Autodesk Inventor part; units mm, degrees
ref_plane "YZ Plane" through (0, 0, 0) normal (1, 0, 0) x (0, 1, 0)
ref_plane "XZ Plane" through (0, 0, 0) normal (0, 1, 0) x (-1, 0, 0)
ref_plane "XY Plane" through (0, 0, 0) normal (0, 0, 1) x (1, 0, 0)
sketch "Esboço1" plane through (0, 0, 0) normal (0, 1, 0) x (-1, 0, 0)
  line L0 (-1.5, -2.5981) -> (1.5, -2.5981)
  line L1 (-1.5, 2.5981) -> (1.5, 2.5981)
  line L2 (1.5, 2.5981) -> (3, 0)
  line L3 (1.5, -2.5981) -> (3, 0)
  line L4 (-1.5, 2.5981) -> (-3, 0)
  line L5 (-3, 0) -> (-1.5, -2.5981)
  point P0 (0, 0)
  dimension "d8" = 3
  dimension "d10" = 3
  dimension "d11" = 3
  dimension "d12" = 3
  dimension "d15" = 1.5
  dimension "d16" = 1.5
  dimension "d17" = 120
  dimension "d18" = 120
  dimension "d19" = 120
  dimension "d20" = 120
  dimension "d21" = 120
  dimension "d22" = 2.5981
extrude "Extrusão1" add sketch "Esboço1" along normal blind 10
sketch "Esboço2" plane through (0, 10, 0) normal (0, 1, 0) x (1, 0, 0)
  circle A0 centre (0, 0) radius 1.25
  dimension "d26" = 2.5
extrude "Extrusão2" add sketch "Esboço2" along normal blind 8
thread "Rosca1"
sketch "Esboço3" plane through (0, 0, 0) normal (0, -1, 0) x (1, 0, 0)
  circle A0 centre (0, 0) radius 1.25
  dimension "d33" = 2.5
extrude "Extrusão3" cut sketch "Esboço3" against normal blind 6
thread "Rosca3"
equation "\"d8\" = 2 * d16"
equation "\"d10\" = 2 * d15"
equation "\"d17\" = d18"
equation "\"d19\" = d18"
equation "\"d20\" = d18"
equation "\"d21\" = d18"
properties part number "Espacador_Placas" material "Alumínio 6061"
Design review of the part built by this model. Coordinates are the model's own, in mm. A direction names the side the tool comes from. Round coordinates to 2 decimals unless told otherwise and drop trailing zeros. Write each loop counter-clockwise with the first axis right and the second up, starting at its lowest first coordinate (ties: lowest second). Pieces come first, ordered by that corner, then holes. Notation, with made-up numbers: (-40, -0.75) - (5, -0.75) arc R22 ccw to (5, 6.25) - close; hole circle Ø8 at (33, 21.25). An arc over 180 degrees is marked (long way). Use a Markdown table: item, result. Add a question column.
1. We need section B-B (z = -0.2). State the section outline as (x, y) points.
2. We need section A-A (x = 0). State the section outline as (y, z) points, then the cut area to 3 significant figures.
3. Mouldability with a two-part tool opening along Z and no side actions: class faces 4 (the face through (2.24, 4.93, 1.32)), 5 (the face through (0, 6, 0)), 6 (the face through (-0.27, 13.94, -1.22)) as +Z half, -Z half, draft (parallel to the pull), parting line (faces both ways), or undercut.
4. For faces 1 (the face through (-1, 0, -1)), 2 (the face through (-1, 10, -1)), 3 (the face through (-0.27, 2.96, -1.22)), list the 3-axis set-ups (+Z, -Z, +X, -X, +Y, -Y) from which the entire face can be reached by the end or side of a thin tool; tool diameter is ignored.
5. We need section C-C (y = 11.5). State the section outline as (x, z) points, then the cut area to 3 significant figures.
6. Clearance check with a flat-ended pin moving along its axis: pin 1 (2 mm diameter, centred on x = 0, z = 0, fed in from -Y). State where the tip first meets the part, or that it passes through.
7. We need section D-D (x = -1.85). State the section outline as (y, z) points, then the cut area to 3 significant figures.
8. Wall thickness on probe 1 along Z at (x, y) = (0, 3.55); probe 2 along Y at (x, z) = (-0.6, 1.9); probe 3 along X at (y, z) = (0.5, -0.05): over which ranges is each line inside the solid? List them lowest first.
Output:
| question | item | result |
|---|---|---|
| 1 | outline | (-2.88, 0) - (-1.23, 0) - (-1.23, 6) - (1.23, 6) - (1.23, 0) - (2.88, 0) - (2.88, 10) - (1.23, 10) - (1.23, 18) - (-1.23, 18) - (-1.23, 10) - (-2.88, 10) - close |
| 2 | outline | (0, -2.6) - (10, -2.6) - (10, -1.25) - (18, -1.25) - (18, 1.25) - (10, 1.25) - (10, 2.6) - (0, 2.6) - (0, 1.25) - (6, 1.25) - (6, -1.25) - (0, -1.25) - close |
| 2 | area | 57.0 mm2 |
| 3 | face 4 | +Z half |
| 3 | face 5 | undercut |
| 3 | face 6 | parting line |
| 4 | face 1 | +Z, -Z, +X, -X, -Y |
| 4 | face 2 | +Y |
| 4 | face 3 | -Y |
| 5 | outline | circle Ø2.5 at (0, 0) |
| 5 | area | 4.91 mm2 |
| 6 | pin 1 | stops at y = 6 |
| 7 | outline | (0, -1.99) - (10, -1.99) - (10, 1.99) - (0, 1.99) - close |
| 7 | area | 39.8 mm2 |
| 8 | probe 1 | z = -2.6 to -1.25, 1.25 to 2.6 |
| 8 | probe 2 | y = 0 to 10 |
| 8 | probe 3 | x = -2.97 to -1.25, 1.25 to 2.97 |
